from build123d import *

# Parameters (mm, degrees)
F0_W           = 93
F0_H           = 17
F1_DEPTH       = 5
F2_D           = 2
F3_D           = 3
F3_CSINK_D     = 5.5
F3_CSINK_ANGLE = 90
F4_R           = 2


with BuildPart() as f1:
    # F0 (on Top) → F1 (new body)
    with BuildSketch(Plane.XY):
        Rectangle(F0_W, F0_H)
    extrude(amount=F1_DEPTH)

    # F2 (through all)
    with Locations(Plane(origin=(0, 0, 0), x_dir=(1, 0, 0), z_dir=(0, 0, -1))):
        with Locations((-41.3, -2.25), (-4.1, -2.25), (4.2, -2.25), (41.4, -2.25)):
            Hole(F2_D / 2)

    # F3 (through all)
    with Locations(Plane(origin=(0, 0, 0), x_dir=(1, 0, 0), z_dir=(0, 0, -1))):
        with Locations((29, -2.25), (-28.9, -2.25)):
            CounterSinkHole(F3_D / 2, F3_CSINK_D / 2, counter_sink_angle=F3_CSINK_ANGLE)

    # F4
    f4_edges = [f1.edges().sort_by_distance(p)[0] for p in [
        (46.5, 8.5, 2.5),
        (46.5, -8.5, 2.5),
        (-46.5, 8.5, 2.5),
        (-46.5, -8.5, 2.5),
    ]]
    fillet(f4_edges, radius=F4_R)


solid = f1.part
Build history of the part. All positions in model axes, mm. Coordinates: 2 decimals unless noted, no trailing zeros. Order: outer loops, then holes, each group sorted by start corner. A loop starts at its lowest first (then second) coordinate and runs counter-clockwise, first axis right, second up. Notation, with made-up numbers: (65, 71.25) - (115, 71.25) arc R20 cw to (115, 95.25) - close; hole circle Ø8 at (42, 69.5). An arc over 180 degrees is marked (long way). Write item = value, one per line. Start each with the question number.
1) Saw through at B-B on z = 3.4. Write the cut outline in (x, y), then the cut area to 3 significant figures.
2) Saw through at D-D on x = 4.2. Write the cut outline in (y, z), then the cut area to 3 significant figures.
3) Two-plate mould, pull along X, no slides. Class faces 1 (the face through (-46.5, 0, 2)), 2 (the face through (-1, 0, 0)), 3 (the face through (-3.31, 2.86, 2.53)): pulls with the +X half, pulls with the -X half, needs draft (parallel to the pull), parting line crosses it, or undercut.
4) Saw through at A-A on x = -28.9. Write the cut outline in (y, z), then the cut area to 3 significant figures.
5) Wall check: line 1 along Y through (x, z) = (-28.9, 2.95); line 2 along Y through (x, z) = (4.2, 3.65); line 3 along Z through (x, y) = (-27, 0.5). Give the ranges that are in metal, low to high. Write a range as from..to.
6) Flat gauge pin, fed straight in: pin 1 Ø5 at (x, y) = (29, 2.25) entering from -Z. Where does the tip first touch, or does it go through?
7) Saw through at C-C on y = 2.25. Count the separate pieces of the cut face and the enclosed holes in it, then the cut area to 3 significant figures.
From the geometry:
q1.outline = (-46.5, -6.5) arc R2 ccw to (-44.5, -8.5) - (44.5, -8.5) arc R2 ccw to (46.5, -6.5) - (46.5, 6.5) arc R2 ccw to (44.5, 8.5) - (-44.5, 8.5) arc R2 ccw to (-46.5, 6.5) - close; hole circle Ø2 at (-41.3, 2.25); hole circle Ø3 at (-28.9, 2.25); hole circle Ø2 at (-4.1, 2.25); hole circle Ø2 at (4.2, 2.25); hole circle Ø3 at (29, 2.25); hole circle Ø2 at (41.4, 2.25)
q1.area = 1,550 mm^2
q2.outline = (-8.5, 0) - (1.25, 0) - (1.25, 5) - (-8.5, 5) - close; (3.25, 0) - (8.5, 0) - (8.5, 5) - (3.25, 5) - close
q2.area = 75.0 mm^2
q3.face_1 = pulls with the -X half
q3.face_2 = needs draft
q3.face_3 = undercut
q4.outline = (-8.5, 0) - (-0.5, 0) - (0.75, 1.25) - (0.75, 5) - (-8.5, 5) - close; (3.75, 1.25) - (5, 0) - (8.5, 0) - (8.5, 5) - (3.75, 5) - close
q4.area = 68.4 mm^2
q5.line_1 = -8.5..0.75, 3.75..8.5
q5.line_2 = -8.5..1.25, 3.25..8.5
q5.line_3 = 0.17..5
q6.pin_1 = 0.25
q7.separate_pieces = 7
q7.enclosed_holes = 0
q7.area = 392 mm^2
